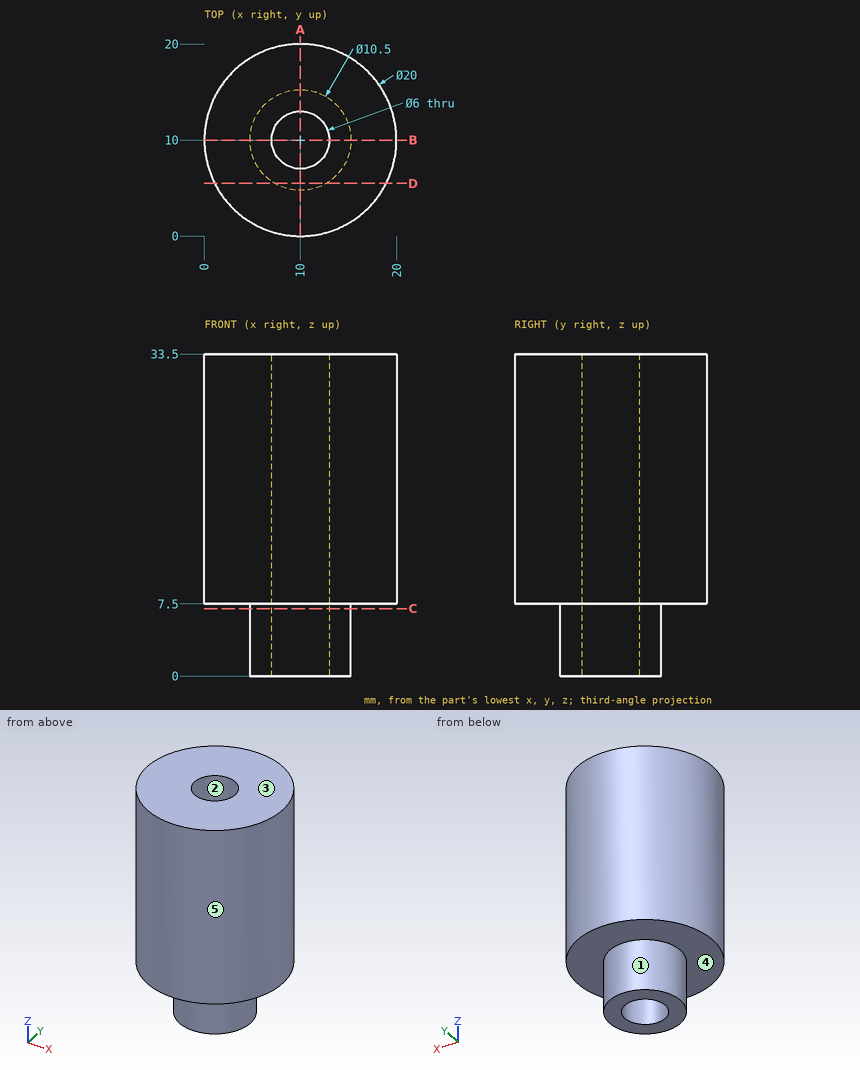
Input: dimensioned drawing with shaded views. Units: mm. Origin: part minimum x, y, z. A direction names the side the tool comes from. Round coordinates to 2 decimals unless told otherwise and drop trailing zeros. Loops run counter-clockwise (first coordinate to the right, second up) from the corner with the lowest first, then second, coordinate; pieces in that order, holes last. Notation, with made-up numbers: (64, 32) -> (90, 32) arc R21 cw to (90, 50) -> close; hole circle Ø2 at (-35, 64.25). An arc over 180 degrees is marked (long way). Answer as a JSON object with one key per item and string values. Group by question number.
Q1. Mould query, pull axis X, two halves, no side actions, for the marked faces 1, 2 and 3. Classes: pulls with the +X half, pulls with the -X half, needs draft (parallel to the pull), parting line crosses it, or undercut.
Q2. Ray query, line 1 (Y direction, x = 10, z = 18); line 2 (Z direction, x = 17.5, y = 8.25); line 3 (Y direction, x = 7.25, z = 3). Return the intervals inside material, ascending. Write a range as from..to.
Q3. Section query A-A (x = 10). Output: boundary loops of the cut face in (y, z), plus the area to 3 significant figures.
Q4. Access query for the marked faces 4 and 5. Directions: +Z, -Z, +X, -X, +Y, -Y. A direction counts if a zero-diameter tool reaches every point of the face in a straight line with its end or side. Return the directions, or none.
Q5. Contact query for flat-ended pins moving along their axis: P1, Ø1.5, axis at y = 8.5, z = 15, coming from the +X side; P2, Ø1.5, axis at x = 7, z = 14.5, coming from the +Y side; P3, Ø3.5, axis at x = 10, y = 10, coming from the -Z side. Output: stop coordinate, or through.
Q6. Section query C-C (z = 7). Output: boundary loops of the cut face in (x, y).
Q7. Section query D-D (y = 5.5). Output: boundary loops of the cut face in (x, z), plus the area to 3 significant figures.
Completed:
{
 "1": {"face 1": "parting line crosses it", "face 2": "undercut", "face 3": "needs draft"},
 "2": {"line 1": "0..7, 13..20", "line 2": "7.5..33.5", "line 3": "5.53..8.8, 11.2..14.47"},
 "3": {"outline": "(0, 7.5) -> (4.75, 7.5) -> (4.75, 0) -> (7, 0) -> (7, 33.5) -> (0, 33.5) -> close; (13, 0) -> (15.25, 0) -> (15.25, 7.5) -> (20, 7.5) -> (20, 33.5) -> (13, 33.5) -> close", "area": "398 mm²"},
 "4": {"face 4": "-Z", "face 5": "+Z, -Z"},
 "5": {"P1": "x = 19.97", "P2": "y = 19.74", "P3": "through"},
 "6": {"outline": "circle Ø10.5 at (10, 10); hole circle Ø6 at (10, 10)"},
 "7": {"outline": "(1.07, 7.5) -> (7.3, 7.5) -> (7.3, 0) -> (12.7, 0) -> (12.7, 7.5) -> (18.93, 7.5) -> (18.93, 33.5) -> (1.07, 33.5) -> close", "area": "505 mm²"}
}
